The model under review builds one solid part; all positions refer to its coordinate system, in mm. Face numbers are marked on the shaded views. Round coordinates to 2 decimals unless told otherwise and drop trailing zeros. Write each loop counter-clockwise with the first axis right and the second up, starting at its lowest first coordinate (ties: lowest second). Pieces come first, ordered by that corner, then holes.
Item 1: Draft analysis for pull direction Z (two halves, no side actions). For the marked faces 1 and 2, state which applies: +Z half, -Z half, draft (parallel to the pull), parting line (faces both ways), or undercut.
Item 2: Add section B-B (z = 2). Give the boundary of the cut face in (x, y), plus the area to 3 significant figures.
Item 3: To check wall thickness, follow L1, parallel to X at y = 1.7, z = 12.5; L2, parallel to X at y = 4.2, z = -5.5; L3, parallel to Z at x = -33.5, y = 4.95. State the ranges of each line that lie inside material, in increasing order.
Item 4: Add section C-C (y = 1). Give the boundary of the cut face in (x, z), plus the area to 3 significant figures.
Item 5: Add section D-D (x = -36.5). Give the boundary of the cut face in (y, z).
Item 6: Clearance check with flat-ended pins moving along their axes: pin 1 Ø2.5 at (x, y) = (45.5, 5) entering from -Z; pin 2 Ø4 at (x, z) = (35.5, -18.5) entering from +Y; pin 3 Ø0.9 at (y, z) = (4, 12) entering from +X. State where each tip first meets the part, or that it passes through.
Item 7: Add section A-A (z = 11). Give the boundary of the cut face in (x, y).
```python
from build123d import *

# Parameters (mm, degrees)
SKETCH2_W           = 180
SKETCH2_H           = 69
BOSS_EXTRUDE1_DEPTH = 3
SKETCH3_W           = 173
SKETCH3_H           = 63
SKETCH3_W_2         = 170
SKETCH3_H_2         = 60
BOSS_EXTRUDE2_DEPTH = 3
SKETCH4_W           = 25.4
SKETCH4_H           = 14
CUT_EXTRUDE1_DEPTH  = 10
SKETCH5_W           = 69
SKETCH5_H           = 1.5
CUT_EXTRUDE2_DEPTH  = 3
SKETCH6_W           = 1.5
SKETCH6_H           = 3.5
CUT_EXTRUDE3_DEPTH  = 3
SKETCH7_R           = 3.5
CUT_EXTRUDE4_DEPTH  = 3
SKETCH8_R           = 32.5
CUT_EXTRUDE5_DEPTH  = 10
SKETCH9_W           = 16
SKETCH9_H           = 16
CUT_EXTRUDE6_DEPTH  = 10
SKETCH10_W          = 72.5
SKETCH10_H          = 8
CUT_EXTRUDE7_DEPTH  = 10
SKETCH11_W          = 7
SKETCH11_H          = 14
CUT_EXTRUDE8_DEPTH  = 10


with BuildPart() as part:
    # Sketch2 → Boss-Extrude1 (new body)
    with BuildSketch(Plane(origin=(0, 0, 0), x_dir=(1, 0, 0), z_dir=(0, 1, 0))):
        Rectangle(SKETCH2_W, SKETCH2_H)
    extrude(amount=BOSS_EXTRUDE1_DEPTH)

    # Sketch3 → Boss-Extrude2 (add)
    with BuildSketch(Plane(origin=(0, 3, 0), x_dir=(1, 0, 0), z_dir=(0, 1, 0))):
        Rectangle(SKETCH3_W, SKETCH3_H)
        Rectangle(SKETCH3_W_2, SKETCH3_H_2, mode=Mode.SUBTRACT)
    extrude(amount=BOSS_EXTRUDE2_DEPTH)

    # Sketch4 → Cut-Extrude1 (cut)
    with BuildSketch(Plane.XZ):
        with Locations((-53.2, 12.5)):
            Rectangle(SKETCH4_W, SKETCH4_H)
    extrude(amount=-CUT_EXTRUDE1_DEPTH, mode=Mode.SUBTRACT)

    # Sketch5 → Cut-Extrude2 (cut)
    with BuildSketch(Plane(origin=(0, 6, 0), x_dir=(1, 0, 0), z_dir=(0, 1, 0))):
        with Locations((52, 30.75)):
            Rectangle(SKETCH5_W, SKETCH5_H)
    extrude(amount=-CUT_EXTRUDE2_DEPTH, mode=Mode.SUBTRACT)

    # Sketch6 → Cut-Extrude3 (cut)
    with BuildSketch(Plane(origin=(0, 6, 0), x_dir=(1, 0, 0), z_dir=(0, 1, 0))):
        with Locations((85.75, 28.25)):
            Rectangle(SKETCH6_W, SKETCH6_H)
    extrude(amount=-CUT_EXTRUDE3_DEPTH, mode=Mode.SUBTRACT)

    # Sketch7 → Cut-Extrude4 (cut)
    with BuildSketch(Plane.XZ):
        Circle(SKETCH7_R)
    extrude(amount=-CUT_EXTRUDE4_DEPTH, mode=Mode.SUBTRACT)

    # Sketch8 → Cut-Extrude5 (cut)
    with BuildSketch(Plane.XZ):
        with Locations((0, 54.5)):
            Circle(SKETCH8_R)
    extrude(amount=-CUT_EXTRUDE5_DEPTH, mode=Mode.SUBTRACT)

    # Sketch9 → Cut-Extrude6 (cut)
    with BuildSketch(Plane.XZ):
        with Locations((0, 22)):
            Rectangle(SKETCH9_W, SKETCH9_H)
    extrude(amount=-CUT_EXTRUDE6_DEPTH, mode=Mode.SUBTRACT)

    # Sketch10 → Cut-Extrude7 (cut)
    with BuildSketch(Plane(origin=(0, 3, 0), x_dir=(1, 0, 0), z_dir=(0, 1, 0))):
        with Locations((53.75, 30.5)):
            Rectangle(SKETCH10_W, SKETCH10_H)
    extrude(amount=-CUT_EXTRUDE7_DEPTH, mode=Mode.SUBTRACT)

    # Sketch11 → Cut-Extrude8 (cut)
    with BuildSketch(Plane(origin=(0, 0, 0), x_dir=(-1, 0, 0), z_dir=(0, -1, 0))):
        with Locations((0, -7)):
            Rectangle(SKETCH11_W, SKETCH11_H)
    extrude(amount=-CUT_EXTRUDE8_DEPTH, mode=Mode.SUBTRACT)


solid = part.part
```
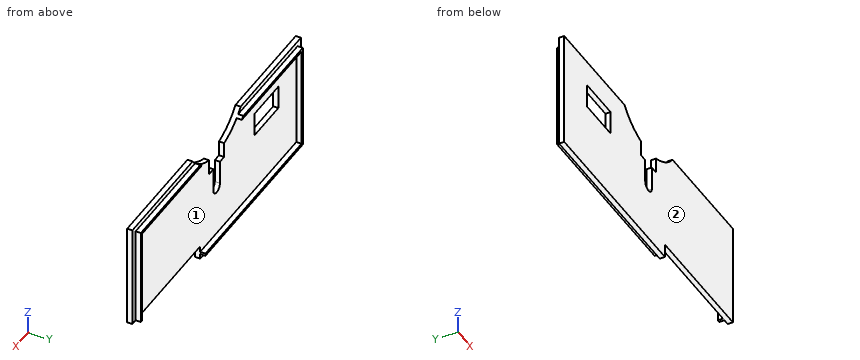
Numbers:
1. face 1: undercut
1. face 2: draft
2. outline: (-90, 0) - (-3.5, 0) - (-3.5, 3) - (-85, 3) - (-85, 6) - (-86.5, 6) - (-86.5, 3) - (-90, 3) - close; (3.5, 0) - (90, 0) - (90, 3) - (86.5, 3) - (86.5, 6) - (85, 6) - (85, 3) - (3.5, 3) - close
2. area: 528 mm2
3. L1: x = -90 to -65.9, -40.5 to -3.5, 3.5 to 90
3. L2: x = -86.5 to -85, 85 to 86.5
3. L3: z = -31.5 to -30, 30 to 31.5
4. outline: (-90, -34.5) - (17.5, -34.5) - (17.5, -26.5) - (90, -26.5) - (90, 34.5) - (25.62, 34.5) arc R32.5 cw to (8, 23) - (8, 14) - (3.5, 14) - (3.5, 0) arc R3.5 cw to (-3.5, 0) - (-3.5, 14) - (-8, 14) - (-8, 23) arc R32.5 cw to (-25.62, 34.5) - (-90, 34.5) - close; hole (-65.9, 5.5) - (-40.5, 5.5) - (-40.5, 19.5) - (-65.9, 19.5) - close
4. area: 10,800 mm2
5. outline: (0, -34.5) - (3, -34.5) - (3, -31.5) - (6, -31.5) - (6, -30) - (3, -30) - (3, 30) - (6, 30) - (6, 31.5) - (3, 31.5) - (3, 34.5) - (0, 34.5) - close
6. pin 1: stops at z = 30
6. pin 2: stops at y = 3
6. pin 3: stops at x = 86.5
7. outline: (-90, 0) - (-65.9, 0) - (-65.9, 3) - (-85, 3) - (-85, 6) - (-86.5, 6) - (-86.5, 3) - (-90, 3) - close; (-40.5, 0) - (-3.5, 0) - (-3.5, 3) - (-40.5, 3) - close; (3.5, 0) - (90, 0) - (90, 3) - (86.5, 3) - (86.5, 6) - (85, 6) - (85, 3) - (3.5, 3) - close
